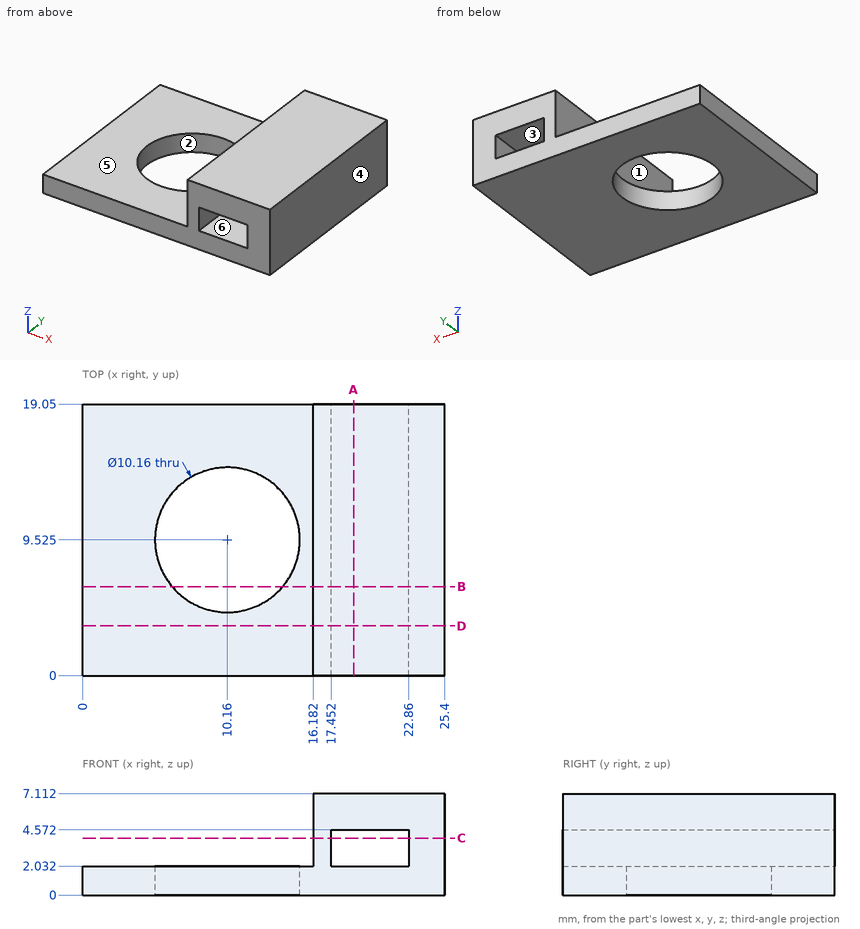
Verification items for this drawing (mm, ordinates from the low corner). A direction names the side the tool comes from. Round coordinates to 2 decimals unless told otherwise and drop trailing zeros. Loops run counter-clockwise (first coordinate to the right, second up) from the corner with the lowest first, then second, coordinate; pieces in that order, holes last. Notation, with made-up numbers: (-23, 70) - (-12, 70) arc R27 ccw to (-12, 90) - close; hole circle Ø8 at (42, 4.25). An arc over 180 degrees is marked (long way). Answer as CSV lines item,"result". Start each with the question number.
Item 1: Set-up check for the marked faces 1, 2 and 3: record each of +Z, -Z, +X, -X, +Y, -Y from which the full face is reachable in a straight line by a thin tool's end or side.
Item 2: Release check for a two-part mould opening along X. For the marked faces 4, 5 and 6 record: +X half, -X half, draft (parallel to the pull), parting line (faces both ways), or undercut.
Item 3: Section check B-B (y = 6.25). Record the boundary of the cut face in (x, z).
Item 4: Section check D-D (y = 3.5). Record the boundary of the cut face in (x, z).
Item 5: Scan lines: line 1 (Z direction, x = 18.75, y = 6); line 2 (Y direction, x = 10.16, z = 0.9) (3 decimals); line 3 (X direction, y = 3.75, z = 3.5). Record each from-to range of solid material in increasing order. Write a range as [from, to].
Item 6: Section check A-A (x = 19). Record the boundary of the cut face in (y, z), and give its area (3 significant figures).
Item 7: Section check C-C (z = 4). Record the boundary of the cut face in (x, y).
Item 8: Depth check by flat-ended pin: P1, Ø6, axis at x = 20.5, y = 5, coming from the -Z side; P2, Ø8, axis at x = 4.5, y = 10.5, coming from the +Z side; P3, Ø2, axis at y = 9, z = 3.5, coming from the -X side. Enter the tip coordinate at first touch or a pass-through.
Report:
1,face 1,"+Z, -X, +Y, -Y"
1,face 2,"+Z, -Z"
1,face 3,"+Y, -Y"
2,face 4,"+X half"
2,face 5,"draft"
2,face 6,"undercut"
3,outline,"(0, 0) - (6.28, 0) - (6.28, 2.03) - (0, 2.03) - close; (14.04, 0) - (25.4, 0) - (25.4, 7.11) - (16.18, 7.11) - (16.18, 2.03) - (14.04, 2.03) - close; hole (17.45, 2.03) - (22.86, 2.03) - (22.86, 4.57) - (17.45, 4.57) - close"
4,outline,"(0, 0) - (25.4, 0) - (25.4, 7.11) - (16.18, 7.11) - (16.18, 2.03) - (0, 2.03) - close; hole (17.45, 2.03) - (22.86, 2.03) - (22.86, 4.57) - (17.45, 4.57) - close"
5,line 1,"z = [0, 2.03], [4.57, 7.11]"
5,line 2,"y = [0, 4.445], [14.605, 19.05]"
5,line 3,"x = [16.18, 17.45], [22.86, 25.4]"
6,outline,"(0, 0) - (19.05, 0) - (19.05, 2.03) - (0, 2.03) - close; (0, 4.57) - (19.05, 4.57) - (19.05, 7.11) - (0, 7.11) - close"
6,area,"87.1 mm2"
7,outline,"(16.18, 0) - (17.45, 0) - (17.45, 19.05) - (16.18, 19.05) - close; (22.86, 0) - (25.4, 0) - (25.4, 19.05) - (22.86, 19.05) - close"
8,P1,"stops at z = 0"
8,P2,"stops at z = 2.03"
8,P3,"stops at x = 16.18"
